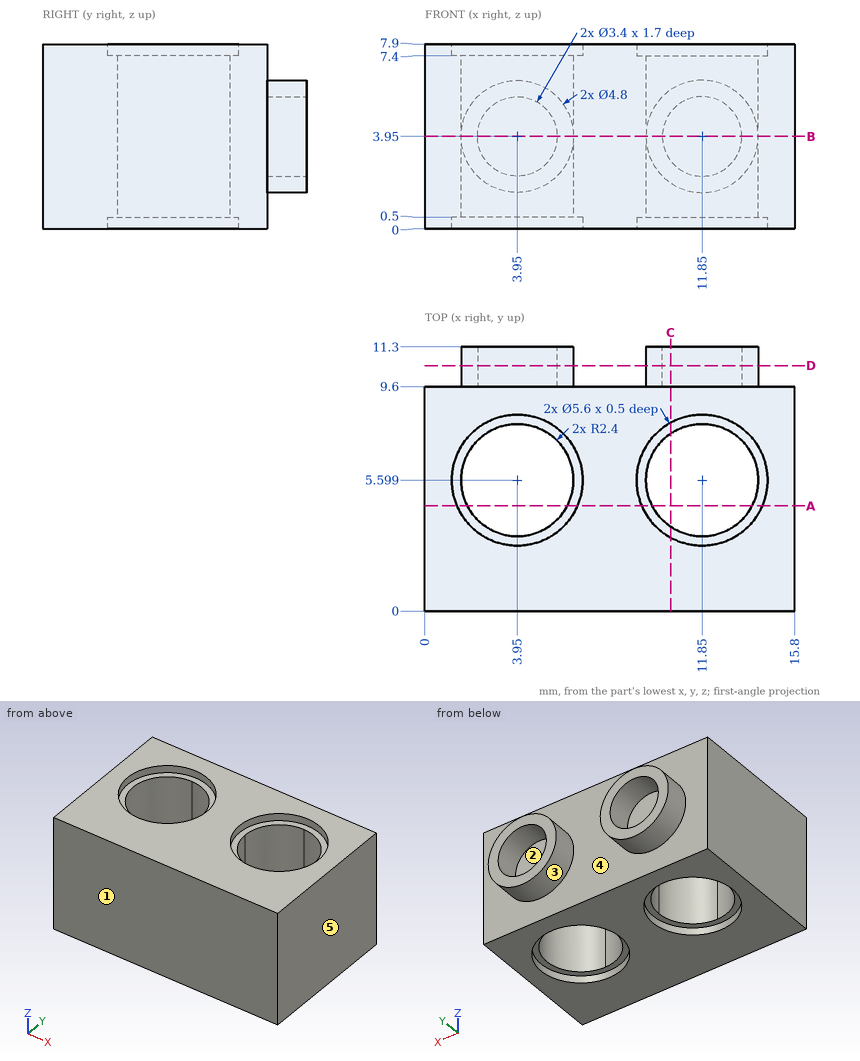
Input: dimensioned drawing with shaded views. Units: mm. Origin: part minimum x, y, z. A direction names the side the tool comes from. Round coordinates to 2 decimals unless told otherwise and drop trailing zeros. Order: outer loops, then holes, each group sorted by start corner. A loop starts at its lowest first (then second) coordinate and runs counter-clockwise, first axis right, second up.
Q1. Section A-A, the plane y = 4.5. Output: boundary loops of the cut face in (x, z) (1 decimal).
Result sheet:
outline: (0, 0) - (1.4, 0) - (1.4, 0.5) - (1.8, 0.5) - (1.8, 7.4) - (1.4, 7.4) - (1.4, 7.9) - (0, 7.9) - close; (6.1, 0.5) - (6.5, 0.5) - (6.5, 0) - (9.3, 0) - (9.3, 0.5) - (9.7, 0.5) - (9.7, 7.4) - (9.3, 7.4) - (9.3, 7.9) - (6.5, 7.9) - (6.5, 7.4) - (6.1, 7.4) - close; (14, 0.5) - (14.4, 0.5) - (14.4, 0) - (15.8, 0) - (15.8, 7.9) - (14.4, 7.9) - (14.4, 7.4) - (14, 7.4) - close
Q2. Access query for the marked faces 4 and 5. Directions: +Z, -Z, +X, -X, +Y, -Y. A direction counts if a zero-diameter tool reaches every point of the face in a straight line with its end or side. Return the directions, or none.
Result sheet:
face 4: +Y
face 5: +Z, -Z, +X, +Y, -Y
Q3. Section C-C, the plane x = 10.5. Output: boundary loops of the cut face in (y, z) (1 decimal), and give its area (3 significant figures).
Result sheet:
outline: (0, 0) - (3.1, 0) - (3.1, 0.5) - (3.6, 0.5) - (3.6, 7.4) - (3.1, 7.4) - (3.1, 7.9) - (0, 7.9) - close; (7.6, 0.5) - (8.1, 0.5) - (8.1, 0) - (9.6, 0) - (9.6, 2) - (11.3, 2) - (11.3, 2.9) - (9.6, 2.9) - (9.6, 5) - (11.3, 5) - (11.3, 5.9) - (9.6, 5.9) - (9.6, 7.9) - (8.1, 7.9) - (8.1, 7.4) - (7.6, 7.4) - close
area: 46.8 mm2
Q4. Material intervals for probe 1 along X at (y, z) = (5.75, 3.5) (1 decimal); probe 2 along Y at (x, z) = (4, 6); probe 3 along X at (y, z) = (7.75, 2) (1 decimal), sorted ascending.
Result sheet:
probe 1: x = 0 to 1.6, 6.3 to 9.5, 14.2 to 15.8
probe 2: y = 0 to 3.2, 8 to 11.3
probe 3: x = 0 to 2.9, 5 to 10.8, 12.9 to 15.8
Q5. Pin query (flat end, axial travel): pin 1 (5 mm diameter, centred on x = 3.95, y = 5.6, fed in from -Z); pin 2 (2.5 mm diameter, centred on x = 3.95, z = 3.95, fed in from +Y); pin 3 (5 mm diameter, centred on x = 11.85, y = 5.6, fed in from +Z); pin 4 (3.5 mm diameter, centred on x = 11.85, y = 5.6, fed in from -Z). Return the tip coordinate at first contact, or that it passes through.
Result sheet:
pin 1: stops at z = 0.5
pin 2: stops at y = 9.6
pin 3: stops at z = 7.4
pin 4: passes through
Q6. Mould query, pull axis Z, two halves, no side actions, for the marked faces 1, 2 and 3. Classes: released by +Z, released by -Z, zero draft, split by the parting line, or undercut.
Result sheet:
face 1: zero draft
face 2: undercut
face 3: split by the parting line
Q7. Section B-B, the plane z = 3.95. Output: boundary loops of the cut face in (x, y).
Result sheet:
outline: (0, 0) - (15.8, 0) - (15.8, 9.6) - (14.25, 9.6) - (14.25, 11.3) - (13.55, 11.3) - (13.55, 9.6) - (10.15, 9.6) - (10.15, 11.3) - (9.45, 11.3) - (9.45, 9.6) - (6.35, 9.6) - (6.35, 11.3) - (5.65, 11.3) - (5.65, 9.6) - (2.25, 9.6) - (2.25, 11.3) - (1.55, 11.3) - (1.55, 9.6) - (0, 9.6) - close; hole circle Ø4.8 at (3.95, 5.6); hole circle Ø4.8 at (11.85, 5.6)
Q8. Section D-D, the plane y = 10.5. Output: boundary loops of the cut face in (x, z).
Result sheet:
outline: circle Ø4.8 at (3.95, 3.95); circle Ø4.8 at (11.85, 3.95); hole circle Ø3.4 at (3.95, 3.95); hole circle Ø3.4 at (11.85, 3.95)
